from build123d import *

# Parameters (mm, degrees)
SKETCH1_R           = 9.525
SKETCH1_R_2         = 2.54
SKETCH1_R_3         = 1.143
BOSS_EXTRUDE1_DEPTH = 6.35
BOSS_EXTRUDE2_DEPTH = 6.35
SKETCH4_R           = 1.143
CUT_EXTRUDE1_DEPTH  = 6.35


with BuildPart() as part:
    # Sketch1 → Boss-Extrude1 (new body)
    with BuildSketch(Plane(origin=(0, 0, 0), x_dir=(1, 0, 0), z_dir=(0, 1, 0))):
        Circle(SKETCH1_R)
        Circle(SKETCH1_R_2, mode=Mode.SUBTRACT)
        with Locations((-5.08, 0)):
            Circle(SKETCH1_R_3, mode=Mode.SUBTRACT)
        with Locations((0, 5.08)):
            Circle(SKETCH1_R_3, mode=Mode.SUBTRACT)
        with Locations((5.08, 0)):
            Circle(SKETCH1_R_3, mode=Mode.SUBTRACT)
        with Locations((0, -5.08)):
            Circle(SKETCH1_R_3, mode=Mode.SUBTRACT)
    extrude(amount=BOSS_EXTRUDE1_DEPTH)

    # Sketch3 → Boss-Extrude2 (add)
    with BuildSketch(Plane(origin=(0, 0, 0), x_dir=(1, 0, 0), z_dir=(0, 1, 0))):
        with BuildLine():
            ThreePointArc((-3.697885259, -8.777885259), (-6.735192091, -6.735192091), (-8.777885259, -3.697885259))
            Line((-8.777885259, -3.697885259), (-71.842048969, -66.762048969))
            Line((-71.842048969, -66.762048969), (-66.762048969, -71.842048969))
            Line((-66.762048969, -71.842048969), (-3.697885259, -8.777885259))
        make_face()
    extrude(amount=BOSS_EXTRUDE2_DEPTH)

    # Sketch4 → Cut-Extrude1 (cut)
    with BuildSketch(Plane(origin=(0, 6.35, 0), x_dir=(1, 0, 0), z_dir=(0, 1, 0))):
        with Locations((-64.821029526, -64.80281229)):
            Circle(SKETCH4_R)
        with Locations((-62.126952689, -62.108735454)):
            Circle(SKETCH4_R)
        with Locations((-52.438602593, -52.489659165)):
            Circle(SKETCH4_R)
        with Locations((-48.846500144, -48.897556717)):
            Circle(SKETCH4_R)
        with Locations((-30.436975096, -30.488031668)):
            Circle(SKETCH4_R)
        with Locations((-26.844872648, -26.89592922)):
            Circle(SKETCH4_R)
    extrude(amount=-CUT_EXTRUDE1_DEPTH, mode=Mode.SUBTRACT)


solid = part.part
The listing builds one solid part. Answer for the finished solid, in the listing's coordinates (mm). Give positions to 0.01 mm unless a question says otherwise; leave off trailing zeros. Loops run counter-clockwise (first coordinate to the right, second up) from the corner with the lowest first, then second, coordinate; pieces in that order, holes last.
Item 1: Find the intervals of material crossed by line 1 along X through (y, z) = (2.5, 0) (3 decimals); line 2 along Z through (x, y) = (-1, 1); line 3 along X through (y, z) = (4.25, 5.08), in increasing order.
Derived:
line 1: x = -9.525 to -6.223, -3.937 to -2.54, 2.54 to 3.937, 6.223 to 9.525
line 2: z = -9.47 to -5.63, -4.53 to -2.33, 2.33 to 4.53, 5.63 to 9.47
line 3: x = -10.16 to -1.14, 1.14 to 8.06
Item 2: Determine the mould class of faces 1 (the flat face through (-25, 0, 25)), 2 (the flat face through (-69.338, 3.131, 69.266)), 3 (the cylindrical face through (3.94, 3.13, -0.05)) for opening direction X: +X half, -X half, draft (parallel to the pull), parting line (faces both ways), or undercut.
Derived:
face 1: draft
face 2: -X half
face 3: undercut
Item 3: A cutting plane is placed at D-D (x = -16). Give the vertices of the cut face in (y, z), then the cut area to 3 significant figures.
Derived:
outline: (0, 10.92) - (6.35, 10.92) - (6.35, 21.08) - (0, 21.08) - close
area: 64.5 mm2
Item 4: A cutting plane is placed at A-A (x = 0). Give the vertices of the cut face in (y, z) (3 decimals), then the cut area to 3 significant figures.
Derived:
outline: (0, -9.525) - (6.35, -9.525) - (6.35, -6.223) - (0, -6.223) - close; (0, -3.937) - (6.35, -3.937) - (6.35, -2.54) - (0, -2.54) - close; (0, 2.54) - (6.35, 2.54) - (6.35, 3.937) - (0, 3.937) - close; (0, 6.223) - (6.35, 6.223) - (6.35, 9.525) - (0, 9.525) - close
area: 59.7 mm2
Item 5: Each of these flat-tipped pins is pushed along its axis until it touches: pin 1 Ø12 at (x, z) = (-58, 47) entering from -Y; pin 2 Ø1.5 at (y, z) = (5, 36.5) entering from +X; pin 3 Ø3 at (x, y) = (-43.5, 5) entering from +Z; pin 4 Ø3 at (y, z) = (5.5, 29) entering from +X. Where does it stop, or does it pass through?
Derived:
pin 1: stops at y = 0
pin 2: stops at x = -30.67
pin 3: stops at z = 50.08
pin 4: stops at x = -22.42
Item 6: A cutting plane is placed at B-B (z = 0). Give the vertices of the cut face in (x, y) (3 decimals), then the cut area to 3 significant figures.
Derived:
outline: (-9.525, 0) - (-6.223, 0) - (-6.223, 6.35) - (-9.525, 6.35) - close; (-3.937, 0) - (-2.54, 0) - (-2.54, 6.35) - (-3.937, 6.35) - close; (2.54, 0) - (3.937, 0) - (3.937, 6.35) - (2.54, 6.35) - close; (6.223, 0) - (9.525, 0) - (9.525, 6.35) - (6.223, 6.35) - close
area: 59.7 mm2
Item 7: A cutting plane is placed at C-C (y = 1.5). Give the number of separate pieces and of enclosed holes in the cut face, then the cut area to 3 significant figures.
Derived:
separate pieces: 1
enclosed holes: 11
area: 861 mm2
